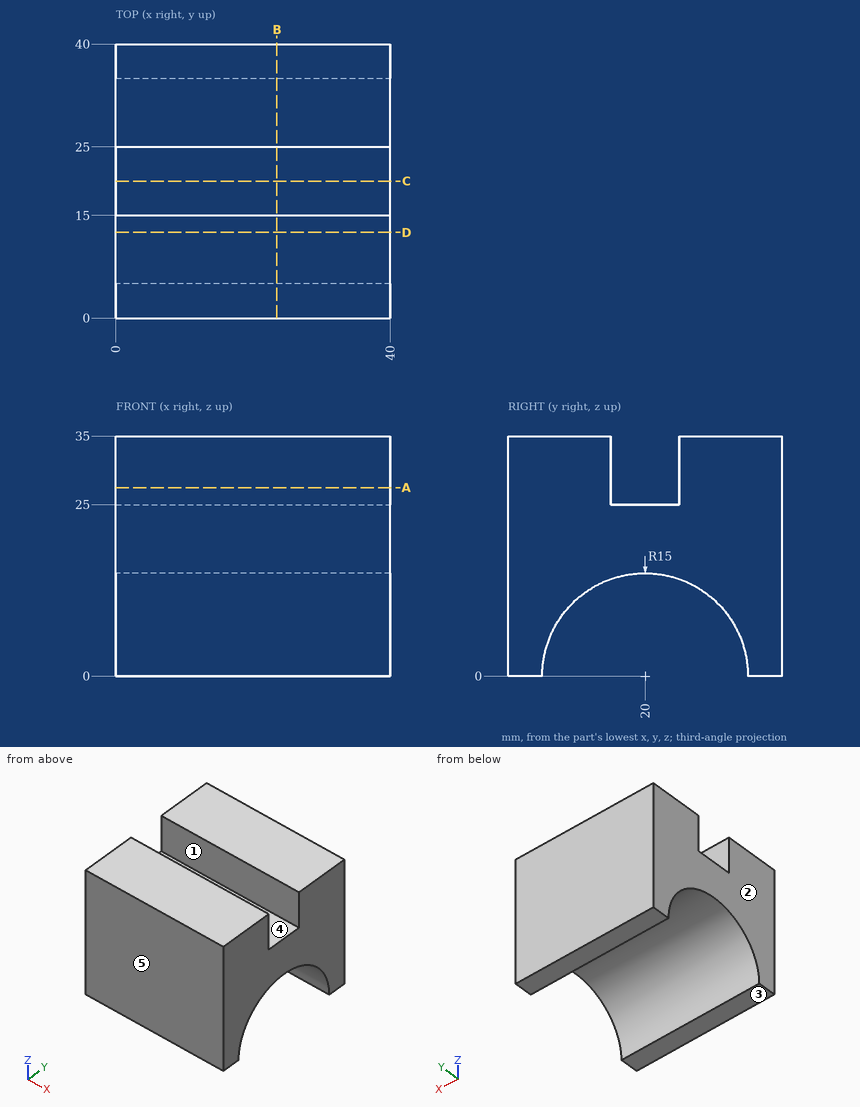
Geometry check sheet. Reference: drawing and pictorial views, mm from the part's lowest x, y, z. A direction names the side the tool comes from. Give positions to 0.01 mm unless a question says otherwise; leave off trailing zeros. Loops run counter-clockwise (first coordinate to the right, second up) from the corner with the lowest first, then second, coordinate; pieces in that order, holes last. Notation, with made-up numbers: M -13,44 L 39,44 A16 cw 39,55 Z; hole C -15,-25.5 d10. An arc over 180 degrees is marked long. One line per question, with ' | ' between items.
Item 1: Thickness scan on line 1 (Y direction, x = 29.5, z = 29.5); line 2 (Y direction, x = 29.5, z = 6.5); line 3 (Z direction, x = 29.5, y = 18). Record the ranges inside material, lowest first. Write a range as [from, to].
Completed:
line 1: y = [0, 15], [25, 40] | line 2: y = [0, 6.48], [33.52, 40] | line 3: z = [14.87, 25]
Item 2: Draft check along Y on the marked faces 3, 4 and 5. Enter one of: +Y half, -Y half, draft (parallel to the pull), parting line (faces both ways), or undercut.
Completed:
face 3: draft | face 4: undercut | face 5: -Y half
Item 3: Section check C-C, the plane y = 20. Record the cut outline in (x, z).
Completed:
outline: M 0,15 L 40,15 L 40,25 L 0,25 Z
Item 4: Section check D-D, the plane y = 12.5. Record the cut outline in (x, z), plus the area to 3 significant figures.
Completed:
outline: M 0,12.99 L 40,12.99 L 40,35 L 0,35 Z | area: 880 mm^2
Item 5: Section check A-A, the plane z = 27.5. Record the cut outline in (x, y), plus the area to 3 significant figures.
Completed:
outline: M 0,0 L 40,0 L 40,15 L 0,15 Z; M 0,25 L 40,25 L 40,40 L 0,40 Z | area: 1,200 mm^2
Item 6: Depth check by flat-ended pin: P1, Ø3, axis at x = 12.5, y = 22, coming from the +Z side; P2, Ø5, axis at x = 6, y = 28.5, coming from the -Z side. Enter the tip coordinate at first touch or a pass-through.
Completed:
P1: stops at z = 25 | P2: stops at z = 10.2
Item 7: Section check B-B, the plane x = 23.5. Record the cut outline in (y, z).
Completed:
outline: M 0,0 L 5,0 A15 cw 35,0 L 40,0 L 40,35 L 25,35 L 25,25 L 15,25 L 15,35 L 0,35 Z
Item 8: Tool access check on the marked faces 1 and 2. Record the directions out of +Z, -Z, +X, -X, +Y, -Y that give a thin tool (end or side, any length) a straight path to the whole face; none if there is none.
Completed:
face 1: +Z, +X, -X | face 2: +Z, -Z, -X, +Y, -Y
